Print and shaded views of the part. All mm, measured from the part's lowest x, y and z. A direction names the side the tool comes from. Round coordinates to 2 decimals unless told otherwise and drop trailing zeros. Loops run counter-clockwise (first coordinate to the right, second up) from the corner with the lowest first, then second, coordinate; pieces in that order, holes last. Notation, with made-up numbers: (53.5, 38) - (85.5, 38) arc R24 ccw to (85.5, 71) - close; hole circle Ø9 at (24.5, -27.75). An arc over 180 degrees is marked (long way). Answer as a JSON object with one key per item and string values.
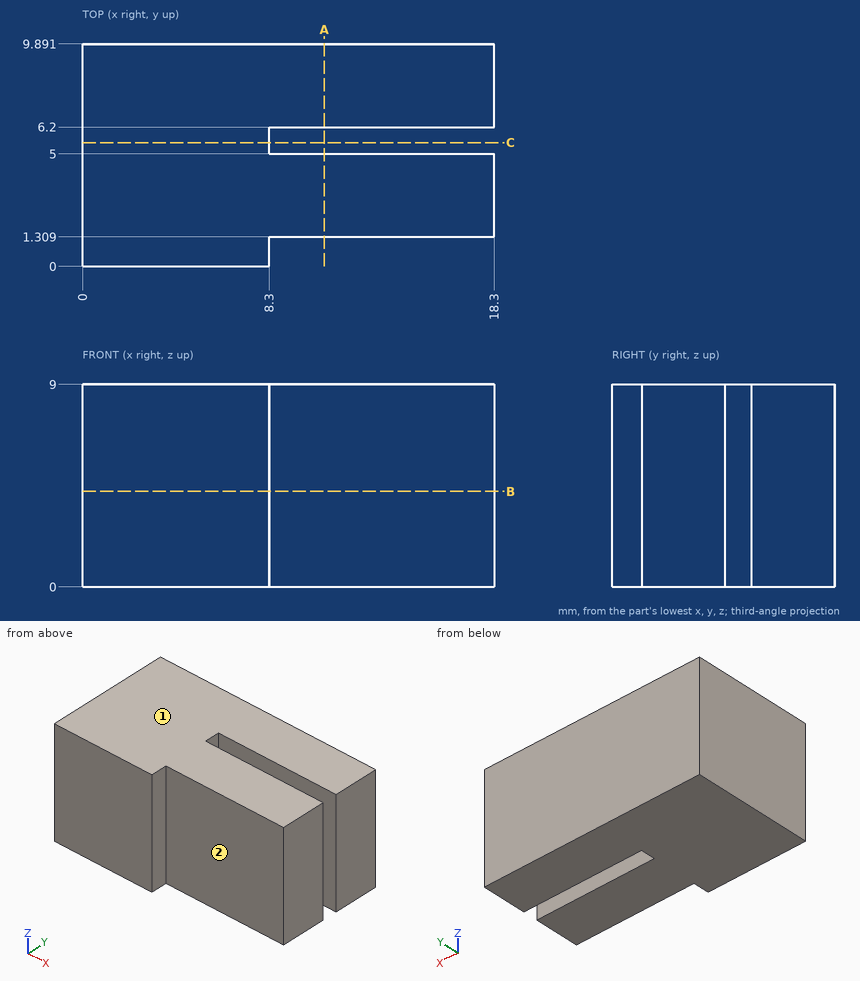
1) Slice it at B-B on z = 4.25. List the corners of the cut face in (x, y), then the cut area to 3 significant figures.
Values follow:
{"outline": "(0, 0) - (8.3, 0) - (8.3, 1.31) - (18.3, 1.31) - (18.3, 5) - (8.3, 5) - (8.3, 6.2) - (18.3, 6.2) - (18.3, 9.89) - (0, 9.89) - close", "area": "156 mm²"}
2) Tool access for the marked faces 1 and 2: list every direction of +Z, -Z, +X, -X, +Y, -Y with a clear straight run to the whole face (end or side of a thin tool).
Values follow:
{"face 1": "+Z, +X, -X, +Y, -Y", "face 2": "+Z, -Z, +X, -Y"}
3) Drop flat-ended pins along their axis: P1, Ø1, axis at y = 0.5, z = 6.5, coming from the +X side; P2, Ø4.5, axis at x = 14.5, z = 3.5, coming from the -Y side. Give the stop position or say it passes through.
Values follow:
{"P1": "x = 8.3", "P2": "y = 1.31"}
4) Probe probe 1 along Y at (x, z) = (10.5, 1); probe 2 along X at (y, z) = (6, 8). List the from-to ranges inside material, lowest first.
Values follow:
{"probe 1": "1.31 to 5, 6.2 to 9.89", "probe 2": "0 to 8.3"}
5) Slice it at A-A on x = 10.75. List the corners of the cut face in (y, z).
Values follow:
{"outline": "(1.31, 0) - (5, 0) - (5, 9) - (1.31, 9) - close; (6.2, 0) - (9.89, 0) - (9.89, 9) - (6.2, 9) - close"}
6) Slice it at C-C on y = 5.5. List the corners of the cut face in (x, z), then the cut area to 3 significant figures.
Values follow:
{"outline": "(0, 0) - (8.3, 0) - (8.3, 9) - (0, 9) - close", "area": "74.7 mm²"}
